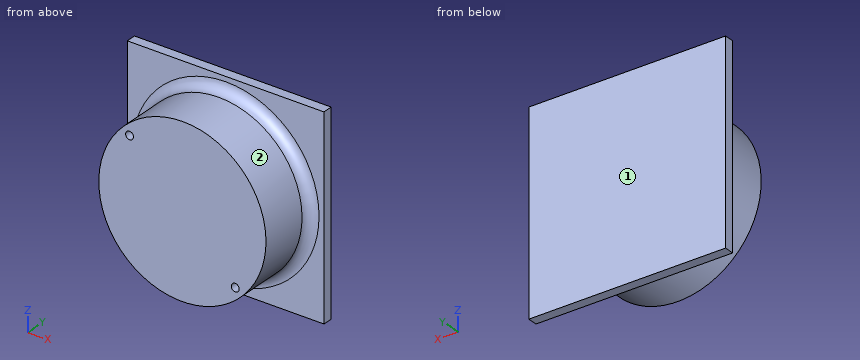
```python
from build123d import *

# Parameters (mm, degrees)
CROQUIS1_R              = 42.5
SALIENTE_EXTRUIR1_DEPTH = 30
CROQUIS2_W              = 100
CROQUIS2_H              = 100
SALIENTE_EXTRUIR2_DEPTH = 5
REDONDEO1_R             = 5
CROQUIS3_R              = 2
CORTAR_EXTRUIR1_DEPTH   = 20


with BuildPart() as part:
    # Croquis1 → Saliente-Extruir1 (new body)
    with BuildSketch(Plane(origin=(0, 0, 0), x_dir=(1, 0, 0), z_dir=(0, 1, 0))):
        with Locations(Location((0, 0, 0), (0, 0, 270))):
            Circle(CROQUIS1_R)
    extrude(amount=SALIENTE_EXTRUIR1_DEPTH)

    # Croquis2 → Saliente-Extruir2 (add)
    with BuildSketch(Plane(origin=(0, 30, 0), x_dir=(1, 0, 0), z_dir=(0, 1, 0))):
        Rectangle(CROQUIS2_W, CROQUIS2_H)
    extrude(amount=SALIENTE_EXTRUIR2_DEPTH)

    # Redondeo1
    redondeo1_edges = [part.edges().sort_by_distance(p)[0] for p in [
        (0, 30, -42.5),
    ]]
    fillet(redondeo1_edges, radius=REDONDEO1_R)

    # Croquis3 → Cortar-Extruir1 (cut)
    with BuildSketch(Plane.XZ):
        with Locations(Location((-26.870057685, 26.870057685, 0), (0, 0, 270))):
            Circle(CROQUIS3_R)
        with Locations(Location((26.870057685, -26.870057685, 0), (0, 0, 90))):
            Circle(CROQUIS3_R)
    extrude(amount=-CORTAR_EXTRUIR1_DEPTH, mode=Mode.SUBTRACT)


solid = part.part
```
Geometry check sheet. Reference: the model listing, model coordinates, mm. Face numbers are marked on the shaded views. A direction names the side the tool comes from. Give positions to 0.01 mm unless a question says otherwise; leave off trailing zeros. Order: outer loops, then holes, each group sorted by start corner. A loop starts at its lowest first (then second) coordinate and runs counter-clockwise, first axis right, second up.
1. Section check A-A, the plane x = 0. Enter the section's corners in (y, z).
2. Gauge pin test, flat ends, axial feed: pin 1 Ø2 at (x, z) = (-27.5, 27.5) entering from -Y; pin 2 Ø1 at (x, y) = (-13, 7) entering from -Z; pin 3 Ø1.5 at (y, z) = (20, 25.5) entering from +X. Record the tip position at first contact, or that the pin passes through.
3. Access from +Z, -Z, +X, -X, +Y, -Y to the whole of each face (thin tool, end or side, straight path). Record for the marked faces 1 and 2.
4. Section check B-B, the plane z = 0. Enter the section's corners in (x, y), and give its area (3 significant figures).
5. Section check D-D, the plane y = 28.5. Enter the section's corners in (x, z).
6. Thickness scan on L1, parallel to Y at x = 45, z = -22.5; L2, parallel to Z at x = 32, y = 14; L3, parallel to X at y = 22, z = -36.5. Record the ranges inside material, lowest first.
7. Section check C-C, the plane y = 3. Enter the section's corners in (x, z).
Values follow:
1. outline: (0, -42.5) - (25, -42.5) arc R5 cw to (30, -47.5) - (30, -50) - (35, -50) - (35, 50) - (30, 50) - (30, 47.5) arc R5 cw to (25, 42.5) - (0, 42.5) - close
2. pin 1: stops at y = 20
2. pin 2: stops at z = -40.62
2. pin 3: stops at x = 34.55
3. face 1: +Z, -Z, +X, -X, +Y
3. face 2: -Y
4. outline: (-50, 30) - (-47.5, 30) arc R5 cw to (-42.5, 25) - (-42.5, 0) - (42.5, 0) - (42.5, 25) arc R5 cw to (47.5, 30) - (50, 30) - (50, 35) - (-50, 35) - close
4. area: 3,060 mm2
5. outline: circle Ø87.86 at (0, 0)
6. L1: y = 30 to 35
6. L2: z = -27.97 to 27.97
6. L3: x = -21.77 to 21.77
7. outline: circle Ø85 at (0, 0); hole circle Ø4 at (-26.87, 26.87); hole circle Ø4 at (26.87, -26.87)
